Can you work these out from the model? Positions are in its coordinate system, mm. A direction names the side the tool comes from. Give positions to 0.01 mm unless a question says otherwise; leave off trailing zeros. Order: outer loops, then holes, each group sorted by start corner. A loop starts at its lowest first (then second) coordinate and runs counter-clockwise, first axis right, second up.
Autodesk Inventor part; units mm, degrees
ref_plane "Start Plane" through (0, 0, -25.0531) normal (0, 0, 1) x (1, 0, 0)
ref_plane "End Plane" through (0, 0, 829.9354) normal (0, 0, 1) x (1, 0, 0)
ref_plane "Work Plane4" through (25.0146, 0.0173, 829.9326) normal (-0.7052, -0.0005, 0.709) x (0.709, -0.0002, 0.7052)
ref_plane "Start Plane" through (0, 0, -25.0531) normal (0, 0, 1) x (1, 0, 0)
ref_plane "End Plane" through (0, 0, 829.9354) normal (0, 0, 1) x (1, 0, 0)
sketch "Sketch" plane through (0, 0, 0) normal (0, 0, 1) x (1, 0, 0)
  line L0 (-25, -21) -> (-25, 21)
  line L1 (-21, 25) -> (21, 25)
  line L2 (25, 21) -> (25, -21)
  line L3 (21, -25) -> (-21, -25)
  arc A0 (-25, -21) -> (-21, -25) centre (-21, -21) ccw
  arc A1 (25, 21) -> (21, 25) centre (21, 21) ccw
  arc A2 (-21, 25) -> (-25, 21) centre (-21, 21) ccw
  arc A3 (21, -25) -> (25, -21) centre (21, -21) ccw
  arc A4 (-21, 23) -> (-23, 21) centre (-21, 21) ccw
  line L4 (-21, 23) -> (21, 23)
  arc A5 (23, 21) -> (21, 23) centre (21, 21) ccw
  line L5 (23, 21) -> (23, -21)
  arc A6 (21, -23) -> (23, -21) centre (21, -21) ccw
  line L6 (21, -23) -> (-21, -23)
  arc A7 (-23, -21) -> (-21, -23) centre (-21, -21) ccw
  line L7 (-23, -21) -> (-23, 21)
  line L8 (0, 36.1598) -> (0, -36.1598) construction
  line L9 (-36.1598, 0) -> (36.1598, 0) construction
  dimension "d7" = 4
  dimension "d9" = 50
  dimension "d11" = 50
  dimension "d12" = 2
  dimension "d15" = 25
  dimension "d16" = 25
extrude "Body" add sketch "Sketch" along normal up to surface (854.9885 mm away) from surface at -25.0531
sketch "Sketch3" plane through (0, 0, 0) normal (0, 0, 1) x (1, 0, 0)
  line L0 (0, 0) -> (10, 0)
ref_plane "Work Plane3" through (0, 0, 0) normal (0, -1, 0) x (1, 0, 0)
sketch "Sketch4" plane through (0, 0, 0) normal (0, -1, 0) x (1, 0, 0)
  line L0 (-2, -25.0531) -> (12, -25.0531)
  line L1 (-2, 829.9354) -> (12, 829.9354)
  dimension "d18" = 854.9885
ref_plane "Work Plane4" through (25.0146, 0.0173, 829.9326) normal (-0.7052, -0.0005, 0.709) x (0.709, -0.0002, 0.7052)
split "Split1" plane through (25.0146, 0.0173, 829.9326) removes the side toward (-0.7052, -0.0005, 0.709)
ref_plane "Work Plane5" through (25.1821, -0.2206, -25.0183) normal (-0.7048, 0.0062, -0.7094) x (-0.7093, 0.015, 0.7048)
split "Split2" plane through (25.1821, -0.2206, -25.0183) removes the side toward (-0.7048, 0.0062, -0.7094)
sketch "Sketch5" plane through (25, -21, 829.9036) normal (1, 0, 0) x (0, 0, -1)
  line L0 (-0.029, 42) -> (0, 0)
  line L1 (-0.0145, 21) -> (189.971, 21)
  line L2 (1.9604, 42) -> (852.5696, 42)
  line L3 (69.971, 42) -> (69.971, -0.006)
  line L4 (806.8722, 42) -> (47.7162, 42)
  line L5 (189.971, 42) -> (189.971, -0.0802)
  point P0 (829.9036, 21)
  point P1 (69.971, 20.997)
  dimension "d19" = 70
  dimension "d20" = 120
hole "Hole1" at (25, 0, 639.9326) at (25, -0.003, 759.9326) direction (-1, 0, 0) diameter 16 depth 50
equation "\"d7\" = G_IR"
equation "\"d9\" = G_W"
equation "\"d11\" = G_H"
equation "\"d12\" = G_T"
equation "\"d15\" = 0.5 * d9"
equation "\"d16\" = 0.5 * d11"
equation "\"d3\" = G_L"
equation "\"G_W\" = 50"
equation "\"G_H\" = 50"
equation "\"G_T\" = 2"
equation "\"G_IR\" = 4"
equation "\"G_L\" = d18"
equation "\"G_OFFSET_START\" = 25.05309"
equation "\"G_OFFSET_END\" = 24.88452"
equation "\"d13\" = -G_OFFSET_START"
equation "\"d14\" = G_OFFSET_END + B_L"
equation "\"B_L\" = 805.05086"
properties part number "ISO 10799-2 - 50x50x2 - 854.99"
1) Which directions (+Z, -Z, +X, -X, +Y, -Y) give clear straight access to the entire face, cutting with the end or side of a thin tool? Please do faces 4 (the face through (0, -23, 397)), 5 (the face through (-24.014, -0.352, 647.925)).
2) Suppose I cut it at C-C (z = 252). Please give me the cut outline in (x, y).
3) Suppose I cut it at A-A (x = -6). Please give me the cut outline in (y, z), and give its area (3 significant figures).
4) If I drill on line 1 (Y direction, x = -10.5, z = 515); line 2 (Y direction, x = 22, z = 697.5), over which ranges is the centre line in solid material (lowest first)?
5) We'd pull the mould along X, two halves only. Please class faces 1 (the face through (-23, 0, 397)), 2 (the face through (23.986, -0.355, 767.925)), 3 (the face through (25, 0, 396)): +X half, -X half, draft (parallel to the pull), parting line (faces both ways), or undercut.
6) Suppose I cut it at B-B (z = 639). Please give me the cut outline in (x, y).
Results:
1. face 4: +Z, -Z
1. face 5: +X, -X
2. outline: (-25, -21) arc R4 ccw to (-21, -25) - (21, -25) arc R4 ccw to (25, -21) - (25, 21) arc R4 ccw to (21, 25) - (-21, 25) arc R4 ccw to (-25, 21) - close; hole (-23, -21) arc R2 ccw to (-21, -23) - (21, -23) arc R2 ccw to (23, -21) - (23, 21) arc R2 ccw to (21, 23) - (-21, 23) arc R2 ccw to (-23, 21) - close
3. outline: (-25, 5.75) - (-23, 5.76) - (-23, 799.07) - (-25, 799.07) - close; (23, 6.16) - (25, 6.18) - (25, 799.1) - (23, 799.1) - close
3. area: 3,170 mm2
4. line 1: y = -25 to -23, 23 to 25
4. line 2: y = -24.87 to -22.73, 22.73 to 24.87
5. face 1: undercut
5. face 2: draft
5. face 3: +X half
6. outline: (-25, -21) arc R4 ccw to (-21, -25) - (21, -25) arc R4 ccw to (25, -21) - (25, -7.95) - (23, -7.95) - (23, -21) arc R2 cw to (21, -23) - (-21, -23) arc R2 cw to (-23, -21) - (-23, -7.95) - (-25, -7.95) - close; (-25, 7.95) - (-23, 7.95) - (-23, 21) arc R2 cw to (-21, 23) - (21, 23) arc R2 cw to (23, 21) - (23, 7.95) - (25, 7.95) - (25, 21) arc R4 ccw to (21, 25) - (-21, 25) arc R4 ccw to (-25, 21) - close
